Answer from the drawing. Dimensions are ordinates in mm from the lowest x, y and z of the part. Round coordinates to 2 decimals unless told otherwise and drop trailing zeros. Write each loop counter-clockwise with the first axis right and the second up, starting at its lowest first coordinate (ties: lowest second). Pieces come first, ordered by that corner, then holes. Notation, with made-up numbers: (21, 26) -> (33, 26) arc R27 cw to (33, 60) -> close; hole circle Ø2 at (-14.75, -20). An arc over 180 degrees is marked (long way). Return JSON: item names as keys, results as strings. Group by question number.
(1) Straight lines are drawn through the part: line 1 (Z direction, x = 40, y = 12.5); line 2 (Z direction, x = 180, y = 7); line 3 (X direction, y = 11.75, z = 14.5) (1 decimal). For each, find the intervals that lie inside material, in ascending order.
(2) A cutting plane is placed at C-C on x = 40. Give the vertices of the cut face in (y, z).
(3) A cutting plane is placed at D-D on x = 95. Give the vertices of the cut face in (y, z), then the cut area to 3 significant figures.
(4) A cutting plane is placed at A-A on y = 12.5. Give the vertices of the cut face in (x, z), then the cut area to 3 significant figures.
(5) Given pin 1 (9 mm diameter, centred on x = 150, z = 15, fed in from +Y); pin 2 (6.5 mm diameter, centred on x = 10, z = 15, fed in from -Y), each flat-ended and moving along its own axis, determine where each tip first touches the part or whether it passes through.
(6) A cutting plane is placed at B-B on z = 15. State how many separate pieces and enclosed holes the cut face has, then the cut area to 3 significant figures.
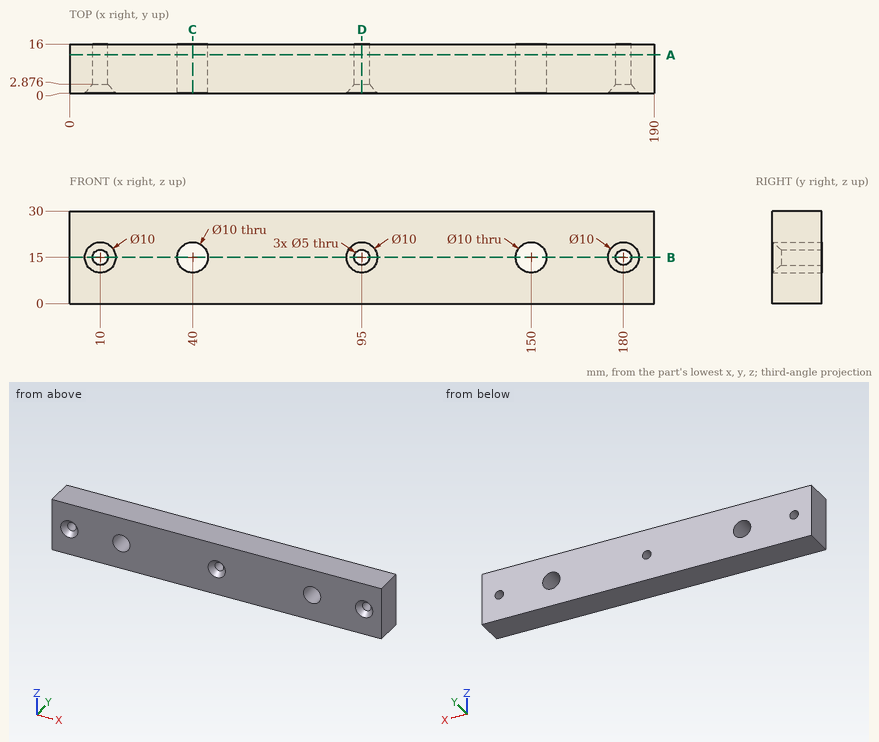
Checks:
{
 "1": {"line 1": "z = 0 to 10, 20 to 30", "line 2": "z = 0 to 12.5, 17.5 to 30", "line 3": "x = 0 to 7.6, 12.4 to 35, 45 to 92.6, 97.4 to 145, 155 to 177.6, 182.4 to 190"},
 "2": {"outline": "(0, 0) -> (16, 0) -> (16, 10) -> (0, 10) -> close; (0, 20) -> (16, 20) -> (16, 30) -> (0, 30) -> close"},
 "3": {"outline": "(0, 0) -> (16, 0) -> (16, 12.5) -> (2.88, 12.5) -> (0, 10) -> close; (0, 20) -> (2.88, 17.5) -> (16, 17.5) -> (16, 30) -> (0, 30) -> close", "area": "393 mm^2"},
 "4": {"outline": "(0, 0) -> (190, 0) -> (190, 30) -> (0, 30) -> close; hole circle Ø5 at (10, 15); hole circle Ø10 at (40, 15); hole circle Ø5 at (95, 15); hole circle Ø10 at (150, 15); hole circle Ø5 at (180, 15)", "area": "5,480 mm^2"},
 "5": {"pin 1": "passes through", "pin 2": "stops at y = 2.01"},
 "6": {"separate pieces": "6", "enclosed holes": "0", "area": "2,460 mm^2"}
}
